Here's how the part is built. I have some questions about the finished solid (model axes, mm). A direction names the side the tool comes from. Round coordinates to 2 decimals unless told otherwise and drop trailing zeros. Order: outer loops, then holes, each group sorted by start corner. A loop starts at its lowest first (then second) coordinate and runs counter-clockwise, first axis right, second up. Notation, with made-up numbers: (58, -18.75) -> (104, -18.75) arc R9 cw to (104, -5.75) -> close; hole circle Ø3 at (5, 46.25). An arc over 180 degrees is marked (long way). One line per item, written item: value.
```python
from build123d import *

# Parameters (mm, degrees)
F0_R            = 63.5
F1_DEPTH        = 25.4
F2_R            = 9.525
F3_DEPTH        = 6.35
F3_COPIES_COUNT = 8
F5_W            = 88.9
F5_H            = 88.9
F6_DEPTH        = 50.8
F4_R            = 19.05
F7_DEPTH        = 101.6
F8_R            = 9.525
F9_DEPTH        = 22.225
F10_R           = 9.525
F11_DEPTH       = 19.05


# Not quite as in the source:
# - a pattern or mirror of a feature is missing from the dataset's text; its kind, count and spacing are read off the source's solid


with BuildPart() as f1:
    # F0 (on Front) → F1 (new body)
    with BuildSketch(Plane.XZ):
        Circle(F0_R)
    extrude(amount=F1_DEPTH)

    # F2 (on face) → F3 (cut)
    with BuildSketch(Plane(origin=(0, 0, 0), x_dir=(-1, 0, 0), z_dir=(0, 1, 0))):
        with Locations((0, 50.8)):
            Circle(F2_R)
    f3 = extrude(amount=-F3_DEPTH, mode=Mode.SUBTRACT)

    # F3_copies: F3 ×8 about axis
    f3_copies_axis = Axis((0, 0, 0), (0, 1, 0))
    for i in range(1, F3_COPIES_COUNT):
        add(f3.rotate(f3_copies_axis, i * 360 / F3_COPIES_COUNT), mode=Mode.SUBTRACT)

    # F5 (on face) → F6 (join)
    with BuildSketch(Plane.XZ.offset(25.4)):
        Rectangle(F5_W, F5_H)
    extrude(amount=F6_DEPTH)

    # F4 (on face) → F7 (cut)
    with BuildSketch(Plane(origin=(0, 0, 0), x_dir=(-1, 0, 0), z_dir=(0, 1, 0))):
        Circle(F4_R)
    extrude(amount=-F7_DEPTH, mode=Mode.SUBTRACT)

    # F8 (on face) → F9 (cut)
    with BuildSketch(Plane.YZ.offset(44.45)):
        with Locations((-60.325, 0)):
            Circle(F8_R)
    extrude(amount=-F9_DEPTH, mode=Mode.SUBTRACT)

    # F10 (on face) → F11 (cut)
    with BuildSketch(Plane(origin=(-44.45, 0, 0), x_dir=(0, -1, 0), z_dir=(-1, 0, 0))):
        with Locations((60.325, 0)):
            Circle(F10_R)
    extrude(amount=-F11_DEPTH, mode=Mode.SUBTRACT)


solid = f1.part
```
Q1. I need wall thicknesses on line 1 along Z through (x, y) = (0, -2) (3 decimals); line 2 along X through (y, z) = (-51.5, -29). Which ranges of each line are inside material? Lowest first, please.
Answers:
line 1: -63.5 to -60.325, -41.275 to -19.05, 19.05 to 41.275, 60.325 to 63.5
line 2: -44.45 to 44.45
Q2. Which directions (+Z, -Z, +X, -X, +Y, -Y) give clear straight access to the entire face, cutting with the end or side of a thin tool? Please do faces 1 (the face through (-44.45, -50, -1)), 2 (the face through (1.24, -3.131, 60.244)), 3 (the face through (4, -25.4, -47)).
Answers:
face 1: +Z, -Z, -X, -Y
face 2: +Y
face 3: -Y
Q3. If we mould it in two halves opening along X, with no side actions, what happens to faces 4 (the face through (-1, -50, 44.45)), 5 (the face through (44.45, -50, -1)), 6 (the face through (31.52, -3.13, 44.37))? For each: pulls with the +X half, pulls with the -X half, needs draft (parallel to the pull), parting line crosses it, or undercut.
Answers:
face 4: needs draft
face 5: pulls with the +X half
face 6: undercut
Q4. For P1, Ø25, axis at x = 0, z = 50.8, coming from the +Y side; P2, Ø6, axis at x = 19.5, y = -41, coming from the +Z side; P3, Ø15, axis at x = -18, y = -44, coming from the -Z side; P4, Ø17, axis at x = 50.8, z = 0, coming from the +Y side, each with a flat end and sliding along its axis, tell me the tip position at first contact or that it passes through.
Answers:
P1: y = 0
P2: z = 44.45
P3: z = -44.45
P4: y = -6.35
Q5. I want a section at A-A on z = 0. Write out the boundary of the cut face in (x, y) (3 decimals).
Answers:
outline: (-63.5, -25.4) -> (-44.45, -25.4) -> (-44.45, -50.8) -> (-25.4, -50.8) -> (-25.4, -69.85) -> (-44.45, -69.85) -> (-44.45, -76.2) -> (-19.05, -76.2) -> (-19.05, 0) -> (-41.275, 0) -> (-41.275, -6.35) -> (-60.325, -6.35) -> (-60.325, 0) -> (-63.5, 0) -> close; (19.05, -76.2) -> (44.45, -76.2) -> (44.45, -69.85) -> (22.225, -69.85) -> (22.225, -50.8) -> (44.45, -50.8) -> (44.45, -25.4) -> (63.5, -25.4) -> (63.5, 0) -> (60.325, 0) -> (60.325, -6.35) -> (41.275, -6.35) -> (41.275, 0) -> (19.05, 0) -> close
Q6. I want a section at C-C on x = 50.8. Write out the boundary of the cut face in (y, z) (3 decimals).
Answers:
outline: (-25.4, -38.1) -> (0, -38.1) -> (0, -9.525) -> (-6.35, -9.525) -> (-6.35, 9.525) -> (0, 9.525) -> (0, 38.1) -> (-25.4, 38.1) -> close
Q7. I want a section at B-B on y = -36.5. Write out the boundary of the cut face in (x, z).
Answers:
outline: (-44.45, -44.45) -> (44.45, -44.45) -> (44.45, 44.45) -> (-44.45, 44.45) -> close; hole circle Ø38.1 at (0, 0)
Q8. I want a section at D-D on z = -50.8. Write out the boundary of the cut face in (x, y) (3 decimals).
Answers:
outline: (-38.1, -25.4) -> (38.1, -25.4) -> (38.1, 0) -> (9.525, 0) -> (9.525, -6.35) -> (-9.525, -6.35) -> (-9.525, 0) -> (-38.1, 0) -> close
